Work out the finished part from the listing and answer in its coordinate system (mm). Give positions to 0.01 mm unless a question says otherwise; leave off trailing zeros. Loops run counter-clockwise (first coordinate to the right, second up) from the corner with the lowest first, then second, coordinate; pieces in that order, holes last. Notation, with made-up numbers: (40, 68.5) - (90, 68.5) arc R16 ccw to (90, 74.5) - close; hole circle Ø10 at (50.5, 35). An arc over 180 degrees is marked (long way). One line per question, with ' | ' between items. Start each with the question number.
1. Each of these flat-tipped pins is pushed along its axis until it touches: pin 1 (1 mm diameter, centred on x = 1.5, y = 3.5, fed in from +Z); pin 2 (3 mm diameter, centred on x = 5, z = -13.5, fed in from +Y). Where does it stop, or does it pass through?
2. Find the intervals of material crossed by line 1 (Y direction, x = 6.25, z = -0.5); line 2 (Y direction, x = 1.9, z = 0); line 3 (Z direction, x = 7.5, y = 0), in increasing order.
3. Section C-C (x = 1.5) is taken. Determine the outline of the cut face in (y, z).
from build123d import *


with BuildPart() as part:
    # Sketch1 → Revolve1 (revolve)
    with BuildSketch(Plane(origin=(0, 0, 0), x_dir=(1, 0, 0), z_dir=(0, 1, 0))):
        with BuildLine():
            Line((7.8, 23.5), (7.8, 22.5))
            Line((7.8, 22.5), (6.842312192, 22.5))
            ThreePointArc((6.842312192, 22.5), (4.871753846, 22.763502242), (3.039661243, 23.535493386))
            Line((3.039661243, 23.535493386), (2.733677959, 23.715483554))
            ThreePointArc((2.733677959, 23.715483554), (2.672608205, 23.741216592), (2.606922927, 23.75))
            Line((2.606922927, 23.75), (0.25, 23.75))
            ThreePointArc((0.25, 23.75), (0.073223305, 23.823223305), (0, 24))
            Line((0, 24), (0, 27.5))
            ThreePointArc((0, 27.5), (0.073223305, 27.676776695), (0.25, 27.75))
            Line((0.25, 27.75), (5.1, 27.75))
            ThreePointArc((5.1, 27.75), (5.276776695, 27.676776695), (5.35, 27.5))
            Line((5.35, 27.5), (5.35, 24.566987298))
            ThreePointArc((5.35, 24.566987298), (5.358518543, 24.502282537), (5.383493649, 24.441987298))
            Line((5.383493649, 24.441987298), (5.410533744, 24.39515248))
            ThreePointArc((5.410533744, 24.39515248), (5.881666372, 23.894323747), (6.526767835, 23.656333252))
            Line((6.526767835, 23.656333252), (7.8, 23.5))
        make_face()
    revolve(axis=Axis((88.99, 0, 0), (-1, 0, 0)))


solid = part.part
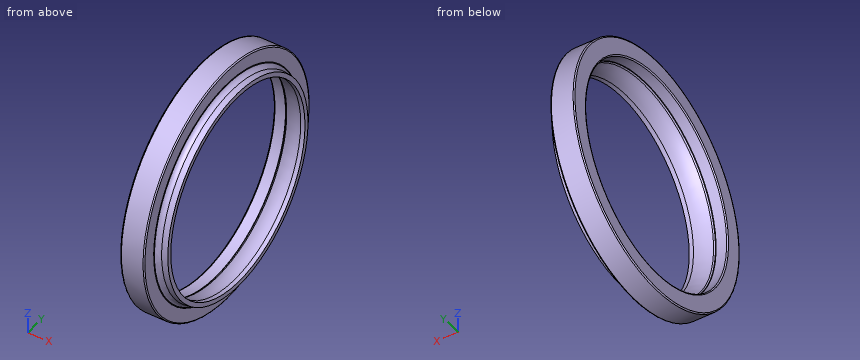
Conclusion:
1) pin 1: z = 27.59 | pin 2: y = 25.02
2) line 1: -23.71 to -22.52, 22.52 to 23.71 | line 2: -27.75 to -23.75, 23.75 to 27.75 | line 3: -23.54 to -22.5, 22.5 to 23.54
3) outline: circle Ø55.5 at (0, 0); hole circle Ø47.5 at (0, 0)
